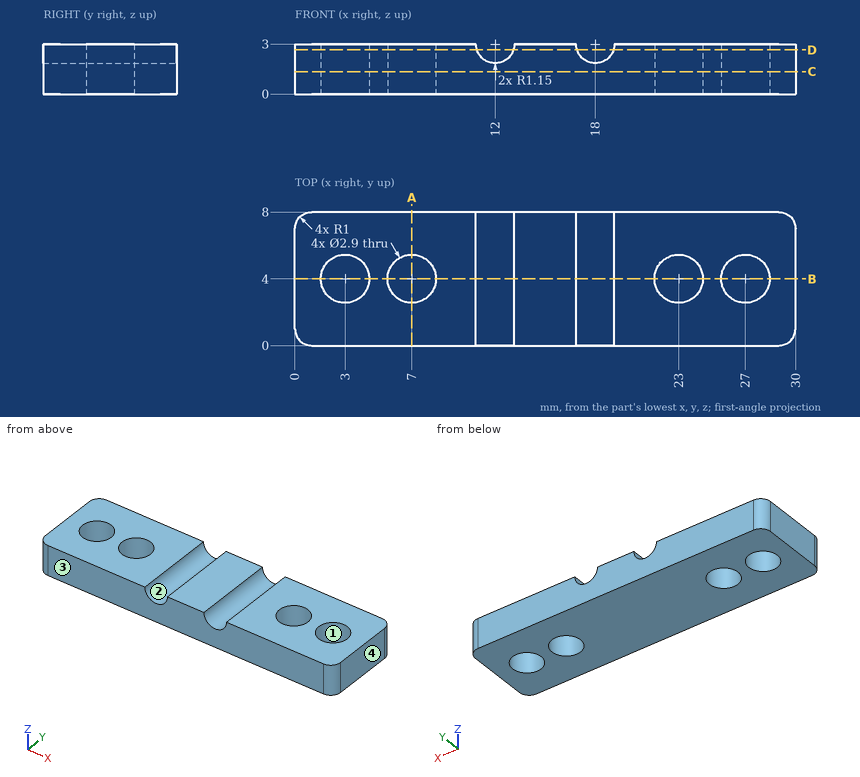
Print and shaded views of the part. All mm, measured from the part's lowest x, y and z. Coordinates: 2 decimals unless noted, no trailing zeros. Loops run counter-clockwise (first coordinate to the right, second up) from the corner with the lowest first, then second, coordinate; pieces in that order, holes last. Notation, with made-up numbers: (-39.5, 56) -> (7.5, 56) arc R22 ccw to (7.5, 82) -> close; hole circle Ø4 at (-2, 2). An arc over 180 degrees is marked (long way). Use a Markdown table: item, result. Add a question column.
Item 1: Pull direction X, two halves, no side cores. Call the marked faces 1, 2, 3 and 4: +X half, -X half, draft (parallel to the pull), parting line (faces both ways), or undercut.
Item 2: Band-saw the part on C-C on z = 1.35. Write the cut outline in (x, y), plus the area to 3 significant figures.
Item 3: Band-saw the part on B-B on y = 4. Write the cut outline in (x, z).
Item 4: Band-saw the part on A-A on x = 7. Write the cut outline in (y, z).
Item 5: Band-saw the part on D-D on z = 2.65. Write the cut outline in (x, y), plus the area to 3 significant figures.
Item 6: Probe probe 1 along Y at (x, z) = (7, 0.95); probe 2 along X at (y, z) = (4.25, 0.65); probe 3 along X at (y, z) = (7, 2.7). List the from-to ranges inside material, lowest first.
Geometry says:
| question | item | result |
|---|---|---|
| 1 | face 1 | undercut |
| 1 | face 2 | undercut |
| 1 | face 3 | draft |
| 1 | face 4 | +X half |
| 2 | outline | (0, 1) arc R1 ccw to (1, 0) -> (29, 0) arc R1 ccw to (30, 1) -> (30, 7) arc R1 ccw to (29, 8) -> (1, 8) arc R1 ccw to (0, 7) -> close; hole circle Ø2.9 at (3, 4); hole circle Ø2.9 at (7, 4); hole circle Ø2.9 at (23, 4); hole circle Ø2.9 at (27, 4) |
| 2 | area | 213 mm² |
| 3 | outline | (0, 0) -> (1.55, 0) -> (1.55, 3) -> (0, 3) -> close; (4.45, 0) -> (5.55, 0) -> (5.55, 3) -> (4.45, 3) -> close; (8.45, 0) -> (21.55, 0) -> (21.55, 3) -> (19.15, 3) arc R1.15 cw to (16.85, 3) -> (13.15, 3) arc R1.15 cw to (10.85, 3) -> (8.45, 3) -> close; (24.45, 0) -> (25.55, 0) -> (25.55, 3) -> (24.45, 3) -> close; (28.45, 0) -> (30, 0) -> (30, 3) -> (28.45, 3) -> close |
| 4 | outline | (0, 0) -> (2.55, 0) -> (2.55, 3) -> (0, 3) -> close; (5.45, 0) -> (8, 0) -> (8, 3) -> (5.45, 3) -> close |
| 5 | outline | (0, 1) arc R1 ccw to (1, 0) -> (10.9, 0) -> (10.9, 8) -> (1, 8) arc R1 ccw to (0, 7) -> close; (13.1, 0) -> (16.9, 0) -> (16.9, 8) -> (13.1, 8) -> close; (19.1, 0) -> (29, 0) arc R1 ccw to (30, 1) -> (30, 7) arc R1 ccw to (29, 8) -> (19.1, 8) -> close; hole circle Ø2.9 at (3, 4); hole circle Ø2.9 at (7, 4); hole circle Ø2.9 at (23, 4); hole circle Ø2.9 at (27, 4) |
| 5 | area | 178 mm² |
| 6 | probe 1 | 0 to 2.55, 5.45 to 8 |
| 6 | probe 2 | 0 to 1.57, 4.43 to 5.57, 8.43 to 21.57, 24.43 to 25.57, 28.43 to 30 |
| 6 | probe 3 | 0 to 10.89, 13.11 to 16.89, 19.11 to 30 |
